Input: part model. Units: mm. Frame: model coordinates. A direction names the side the tool comes from. Round coordinates to 2 decimals unless told otherwise and drop trailing zeros. Loops run counter-clockwise (first coordinate to the right, second up) from the corner with the lowest first, then second, coordinate; pieces in that order, holes last. Notation, with made-up numbers: M 21.25,34.25 L 28.25,34.25 A9 ccw 28.25,42.25 Z; hole C 77,68.25 d4. An arc over 180 degrees is marked long. Put each result on its own line as item: value. Start each with the question number.
1) Pin query (flat end, axial travel): pin 1 (8 mm diameter, centred on y = 31.5, z = 21, fed in from -X); pin 2 (3 mm diameter, centred on y = 33.5, z = 17.5, fed in from +X); pin 3 (10 mm diameter, centred on x = -12, z = -2.5, fed in from +Y); pin 4 (10.5 mm diameter, centred on x = 14, y = 32.5, fed in from -Z). Return the tip coordinate at first contact, or that it passes through.
2) Section A-A on y = 16.5. Output: boundary loops of the cut face in (x, z), plus the area to 3 significant figures.
3) Section D-D on x = -5.5. Output: boundary loops of the cut face in (y, z).
4) Draft query along X for faces 1 (the face through (35, 10, 0)), 2 (the face through (-50, 5, 0)), 3 (the face through (-40, 7, -1)), 4 (the face through (3.95, 34, 19)). Return one class per face: +X half, -X half, draft (parallel to the pull), parting line (faces both ways), or undercut.
5) Section B-B on z = 0. Output: boundary loops of the cut face in (x, y) (3 decimals).
6) Line query: probe 1 along X at (y, z) = (29, 14); probe 2 along X at (y, z) = (1.75, 0) (3 decimals); probe 3 along Y at (x, z) = (-23, 16). Output: solid intervals per line, ascending.
7) Reachability of faces 5 (the face through (-2.5, 36.1, 14.8)), 6 (the face through (42, 10, 6)), 7 (the face through (-1, 7, -25)), 8 (the face through (-1, 29, 19)), 9 (the face through (-43, 10, 6)) from +Z, -Z, +X, -X, +Y, -Y: full face, straight path, thin tool, end or side. Return the list, or none.
8) Section C-C on y = 32.5. State how many separate pieces and enclosed holes the cut face has, plus the area to 3 significant figures.
from build123d import *

# Parameters (mm, degrees)
SKETCH1_W           = 100
SKETCH1_H           = 50
BOSS_EXTRUDE1_DEPTH = 15
SKETCH2_W           = 30
SKETCH2_H           = 12
CUT_EXTRUDE1_DEPTH  = 8
SKETCH7_W           = 23
SKETCH7_H           = 12
BOSS_EXTRUDE2_DEPTH = 10
SKETCH8_W           = 2.95
SKETCH8_H           = 12
BOSS_EXTRUDE3_DEPTH = 20
SKETCH10_R          = 1.5
CUT_EXTRUDE2_DEPTH  = 50
FILLET1_R           = 1.5
FILLET2_R           = 1
SKETCH11_R          = 1.975
CUT_EXTRUDE3_DEPTH  = 20
SKETCH12_R          = 1.975
CUT_EXTRUDE4_DEPTH  = 20


with BuildPart() as part:
    # Sketch1 → Boss-Extrude1 (new body)
    with BuildSketch(Plane(origin=(0, 0, 0), x_dir=(1, 0, 0), z_dir=(0, 1, 0))):
        Rectangle(SKETCH1_W, SKETCH1_H)
    extrude(amount=BOSS_EXTRUDE1_DEPTH)

    # Sketch2 → Cut-Extrude1 (cut)
    with BuildSketch(Plane(origin=(0, 15, 0), x_dir=(1, 0, 0), z_dir=(0, 1, 0))):
        with Locations((-50, 0)):
            Rectangle(SKETCH2_W, SKETCH2_H)
        with Locations((50, 0)):
            Rectangle(SKETCH2_W, SKETCH2_H)
    extrude(amount=-CUT_EXTRUDE1_DEPTH, mode=Mode.SUBTRACT)

    # Sketch7 → Boss-Extrude2 (add)
    with BuildSketch(Plane(origin=(0, 15, 0), x_dir=(1, 0, 0), z_dir=(0, 1, 0))):
        with Locations((12.5, -19)):
            Rectangle(SKETCH7_W, SKETCH7_H)
    boss_extrude2 = extrude(amount=BOSS_EXTRUDE2_DEPTH)

    # Sketch8 → Boss-Extrude3 (add)
    with BuildSketch(Plane(origin=(0, 25, 0), x_dir=(1, 0, 0), z_dir=(0, 1, 0))):
        with Locations((2.475, -19)):
            Rectangle(SKETCH8_W, SKETCH8_H)
        with Locations((22.525, -19)):
            Rectangle(SKETCH8_W, SKETCH8_H)
    boss_extrude3 = extrude(amount=BOSS_EXTRUDE3_DEPTH)

    # Sketch10 → Cut-Extrude2 (cut, through all)
    with BuildSketch(Plane.ZY.offset(-1)):
        with Locations((16, 37)):
            Circle(SKETCH10_R)
        with Locations((22, 37)):
            Circle(SKETCH10_R)
    cut_extrude2 = extrude(amount=-CUT_EXTRUDE2_DEPTH, mode=Mode.SUBTRACT)

    # Mirror1: Boss-Extrude2, Boss-Extrude3, Cut-Extrude2 across plane
    add(boss_extrude2.mirror(Plane(origin=(0, 0, 0), x_dir=(0, 0, 1), z_dir=(1, 0, 0))))
    add(boss_extrude3.mirror(Plane(origin=(0, 0, 0), x_dir=(0, 0, 1), z_dir=(1, 0, 0))))
    add(cut_extrude2.mirror(Plane(origin=(0, 0, 0), x_dir=(0, 0, 1), z_dir=(1, 0, 0))), mode=Mode.SUBTRACT)

    # Fillet1
    fillet1_edges = [part.edges().sort_by_distance(p)[0] for p in [
        (-12.5, 25, 25),
        (-12.5, 25, 13),
        (-50, 15, -15.5),
        (50, 15, -15.5),
        (-50, 15, 15.5),
        (42.5, 15, -6),
        (-37, 15, 25),
        (-42.5, 15, 6),
        (-50, 7, 0),
        (50, 7, 0),
        (-35, 15, 0),
        (-42.5, 15, -6),
        (42.5, 15, 6),
        (35, 15, 0),
        (50, 15, 15.5),
        (37, 15, 25),
        (12.5, 25, 25),
        (12.5, 25, 13),
        (50, 7.5, 25),
        (-50, 7.5, 25),
        (-50, 7.5, -25),
        (50, 7.5, -25),
        (0, 15, -25),
    ]]
    fillet(fillet1_edges, radius=FILLET1_R)

    # Fillet2
    fillet2_edges = [part.edges().sort_by_distance(p)[0] for p in [
        (-24, 30, 13),
        (-24, 30, 25),
        (-1, 30, 25),
        (-1, 30, 13),
        (-3.95, 45, 19),
        (-3.95, 35, 13),
        (-3.95, 35, 25),
        (-1, 45, 19),
        (-21.05, 35, 13),
        (-24, 45, 19),
        (-21.05, 45, 19),
        (-21.05, 35, 25),
        (24, 30, 25),
        (24, 30, 13),
        (1, 30, 13),
        (1, 30, 25),
        (3.95, 35, 13),
        (3.95, 35, 25),
        (1, 45, 19),
        (3.95, 45, 19),
        (21.05, 35, 13),
        (21.05, 35, 25),
        (21.05, 45, 19),
        (24, 45, 19),
    ]]
    fillet(fillet2_edges, radius=FILLET2_R)

    # Sketch11 → Cut-Extrude3 (cut)
    with BuildSketch(Plane(origin=(0, 7, 0), x_dir=(1, 0, 0), z_dir=(0, 1, 0))):
        with Locations((42, 0)):
            Circle(SKETCH11_R)
    extrude(amount=-CUT_EXTRUDE3_DEPTH, mode=Mode.SUBTRACT)

    # Sketch12 → Cut-Extrude4 (cut)
    with BuildSketch(Plane(origin=(0, 7, 0), x_dir=(1, 0, 0), z_dir=(0, 1, 0))):
        with Locations((-42, 0)):
            Circle(SKETCH12_R)
    extrude(amount=-CUT_EXTRUDE4_DEPTH, mode=Mode.SUBTRACT)


solid = part.part
Geometry results:
1. pin 1: stops at x = -24
1. pin 2: stops at x = 24
1. pin 3: stops at y = 15
1. pin 4: passes through
2. outline: M -24,14 A1 ccw -23,13 L -2,13 A1 ccw -1,14 L -1,24 A1 ccw -2,25 L -23,25 A1 ccw -24,24 Z; M 1,14 A1 ccw 2,13 L 23,13 A1 ccw 24,14 L 24,24 A1 ccw 23,25 L 2,25 A1 ccw 1,24 Z
2. area: 550 mm²
3. outline: M 0,-25 L 13.5,-25 A1.5 ccw 15,-23.5 L 15,13 L 23.5,13 A1.5 ccw 25,14.5 L 25,23.5 A1.5 ccw 23.5,25 L 0,25 Z
4. face 1: +X half
4. face 2: -X half
4. face 3: draft
4. face 4: undercut
5. outline: M -50,0 L -43.975,0 L -43.975,7 L -48.5,7 A1.5 ccw -50,5.5 Z; M -40.025,0 L 40.025,0 L 40.025,7 L 35,7 L 35,13.5 A1.5 ccw 33.5,15 L -33.5,15 A1.5 ccw -35,13.5 L -35,7 L -40.025,7 Z; M 43.975,0 L 50,0 L 50,5.5 A1.5 ccw 48.5,7 L 43.975,7 Z
6. probe 1: x = -24 to -21.05, -3.95 to -1, 1 to 3.95, 21.05 to 24
6. probe 2: x = -50 to -43.975, -40.025 to 40.025, 43.975 to 50
6. probe 3: y = 0 to 35.5, 38.5 to 45
7. face 5: +X, -X
7. face 6: +X, +Y
7. face 7: -Z, +X, -X, +Y, -Y
7. face 8: +Z, -Z, +Y
7. face 9: -X, +Y
8. separate pieces: 4
8. enclosed holes: 0
8. area: 138 mm²
